Geometry: final body of the model. Coordinates: model frame, mm. A direction names the side the tool comes from. Give positions to 0.01 mm unless a question says otherwise; leave off trailing zeros. Order: outer loops, then holes, each group sorted by start corner. A loop starts at its lowest first (then second) coordinate and runs counter-clockwise, first axis right, second up. Notation, with made-up numbers: (-20.5, 13.5) -> (-8.5, 13.5) arc R20 ccw to (-8.5, 44.5) -> close; hole circle Ø2 at (-35.5, 1.5). An arc over 180 degrees is marked (long way). Answer in a Markdown table with one row per item. Add a question column.
Q1. Cut plane D-D on z = 1. Return the cut outline in (x, y) (3 decimals), and give its area (3 significant figures).
Q2. Cut plane C-C on y = 4. Return the cut outline in (x, z) (3 decimals).
Q3. Cut plane A-A on y = 17.5. Return the cut outline in (x, z) (3 decimals), and give its area (3 significant figures).
Q4. Contact query for flat-ended pins moving along their axis: P1, Ø4.5, axis at x = 12.5, y = 22, coming from the +Z side; P2, Ø3, axis at y = 18, z = 8.5, coming from the -X side; P3, Ø1.7, axis at x = 12, y = 23.5, coming from the -Z side; P4, Ø3, axis at y = 4, z = 2, coming from the +X side. Output: stop coordinate, or through.
Q5. Set-up query: faces 4 (the face through (11.03, 25, 1.48)), 5 (the face through (9.553, 22.63, 14.021)), 6 (the face through (9, 27.5, 8)), 7 (the face through (10, 29, 15.5)), 8 (the face through (0.6, 21.04, 14.93)). Return all of +Z, -Z, +X, -X, +Y, -Y with unobstructed straight access to the full face (end or side cutting, diameter ignored); none if empty.
Q6. Cut plane B-B on z = 4. Return the cut outline in (x, y), and give its area (3 significant figures).
Q7. Line query: line 1 along Z through (x, y) = (13.5, 10) (3 decimals); line 2 along Y through (x, z) = (12.5, 4.15); line 3 along Y through (x, z) = (3.5, 2). Output: solid intervals per line, ascending. Write a range as from..to.
Q8. Pull-direction query (Z, two-part tool) for faces 1 (the face through (14, 21, 12.5)), 2 (the face through (9, 14, 10.425)), 3 (the face through (1.099, 4, 2)); classes: +Z half, -Z half, draft (parallel to the pull), parting line (faces both ways), or undercut.
from build123d import *

# Parameters (mm, degrees)
PAD_DEPTH       = 15.5
SKETCH001_W     = 27.5
SKETCH001_H     = 5.35
POCKET_DEPTH    = 18.501
SKETCH002_R     = 1.7
POCKET001_DEPTH = 15.501
FILLET_R        = 10
FILLET001_R     = 2
SKETCH003_R     = 2.95
POCKET002_DEPTH = 3
POCKET003_DEPTH = 3


with BuildPart() as part:
    # Sketch → Pad (new body)
    with BuildSketch(Plane.XY):
        with BuildLine():
            Line((18.5, 60), (18.5, 0))
            Line((18.5, 0), (0, 0))
            Line((0, 0), (0, 41.5))
            ThreePointArc((18.5, 60), (5.418525, 54.581475), (0, 41.5))
        make_face()
    extrude(amount=PAD_DEPTH)

    # Sketch001 (on Face1 of Pad) → Pocket (cut, through all)
    with BuildSketch(Plane.YZ.offset(18.5)):
        with Locations((13.75, 7.75)):
            Rectangle(SKETCH001_W, SKETCH001_H)
    extrude(amount=-POCKET_DEPTH, mode=Mode.SUBTRACT)

    # Sketch002 (on Face8 of Pocket) → Pocket001 (cut, through all)
    with BuildSketch(Plane.XY.offset(15.5)):
        with Locations((4, 4)):
            Circle(SKETCH002_R)
        with Locations((12.5, 22.5)):
            Circle(SKETCH002_R)
    extrude(amount=-POCKET001_DEPTH, mode=Mode.SUBTRACT)

    # Fillet
    fillet_edges = [part.edges().sort_by_distance(p)[0] for p in [
        (18.5, 0, 12.9625),
        (18.5, 0, 2.5375),
    ]]
    fillet(fillet_edges, radius=FILLET_R)

    # Fillet001
    fillet001_edges = [part.edges().sort_by_distance(p)[0] for p in [
        (0, 20.75, 15.5),
        (0, 20.75, 0),
    ]]
    fillet(fillet001_edges, radius=FILLET001_R)

    # Sketch003 (on Face9 of Fillet001) → Pocket002 (cut)
    with BuildSketch(Plane.XY.offset(15.5)):
        with Locations((12.5, 22.5)):
            Circle(SKETCH003_R)
        with Locations((4, 4)):
            Circle(SKETCH003_R)
    extrude(amount=-POCKET002_DEPTH, mode=Mode.SUBTRACT)

    # Sketch004 (on Face2 of Pocket002) → Pocket003 (cut)
    with BuildSketch(Plane(origin=(0, 0, 0), x_dir=(1, 0, 0), z_dir=(0, 0, -1))):
        Polygon((12.5, -25.85), (15.401185, -24.175), (15.401185, -20.825), (12.5, -19.15), (9.598815, -20.825), (9.598815, -24.175), align=None)
        Polygon((4, -7.35), (6.901185, -5.675), (6.901185, -2.325), (4, -0.65), (1.098815, -2.325), (1.098815, -5.675), align=None)
    extrude(amount=-POCKET003_DEPTH, mode=Mode.SUBTRACT)


solid = part.part
Completed:
| question | item | result |
|---|---|---|
| 1 | outline | (0.268, 0) -> (8.5, 0) arc R10 ccw to (18.5, 10) -> (18.5, 59.732) arc R18.232 ccw to (0.268, 41.5) -> close; hole (1.099, 2.325) -> (4, 0.65) -> (6.901, 2.325) -> (6.901, 5.675) -> (4, 7.35) -> (1.099, 5.675) -> close; hole (9.599, 20.825) -> (12.5, 19.15) -> (15.401, 20.825) -> (15.401, 24.175) -> (12.5, 25.85) -> (9.599, 24.175) -> close |
| 1 | area | 938 mm² |
| 2 | outline | (0, 2) arc R2 ccw to (1.099, 0.215) -> (1.099, 3) -> (2.3, 3) -> (2.3, 5.075) -> (0, 5.075) -> close; (0, 10.425) -> (2.3, 10.425) -> (2.3, 12.5) -> (1.05, 12.5) -> (1.05, 15.26) arc R2 ccw to (0, 13.5) -> close; (5.7, 3) -> (6.901, 3) -> (6.901, 0) -> (16.5, 0) -> (16.5, 5.075) -> (5.7, 5.075) -> close; (5.7, 10.425) -> (16.5, 10.425) -> (16.5, 15.5) -> (6.95, 15.5) -> (6.95, 12.5) -> (5.7, 12.5) -> close |
| 3 | outline | (0, 2) arc R2 ccw to (2, 0) -> (18.5, 0) -> (18.5, 5.075) -> (0, 5.075) -> close; (0, 10.425) -> (18.5, 10.425) -> (18.5, 15.5) -> (2, 15.5) arc R2 ccw to (0, 13.5) -> close |
| 3 | area | 186 mm² |
| 4 | P1 | stops at z = 12.5 |
| 4 | P2 | passes through |
| 4 | P3 | stops at z = 3 |
| 4 | P4 | stops at x = 17.43 |
| 5 | face 4 | -Z |
| 5 | face 5 | +Z |
| 5 | face 6 | +X, -X, -Y |
| 5 | face 7 | +Z, +X, -X, +Y, -Y |
| 5 | face 8 | +Z, -X, +Y, -Y |
| 6 | outline | (0, 0) -> (8.5, 0) arc R10 ccw to (18.5, 10) -> (18.5, 60) arc R18.5 ccw to (0, 41.5) -> close; hole circle Ø3.4 at (4, 4); hole circle Ø3.4 at (12.5, 22.5) |
| 6 | area | 997 mm² |
| 7 | line 1 | z = 0..5.075, 10.425..15.5 |
| 7 | line 2 | y = 0.83..20.8, 24.2..59 |
| 7 | line 3 | y = 0..0.94, 7.06..52.33 |
| 8 | face 1 | +Z half |
| 8 | face 2 | undercut |
| 8 | face 3 | draft |
